Input: part model. Units: mm. Frame: model coordinates. Give positions to 0.01 mm unless a question says otherwise; leave off trailing zeros. Answer as a JSON object with one key per item and string values. Group by question number.
1) Ray query, L1, parallel to X at y = -0.9, z = -44; L2, parallel to Z at x = 123.5, y = -1.2; L3, parallel to Z at x = 13.5, y = -0.9. Return the intervals inside material, ascending.
2) First-contact query: P1, Ø1, axis at x = 26.5, y = -3.5, coming from the +Z side; P2, Ø1, axis at y = -2.5, z = -38.5, coming from the +X side; P3, Ø2, axis at y = -1.5, z = -44.5, coming from the -X side. Flat tips, straight axial feed; report the tip coordinate or a pass-through.
3) Section query A-A on y = -3.05. Count the separate pieces of the cut face and the enclosed holes in it, plus the area to 3 significant figures.
from build123d import *

# Parameters (mm, degrees)
F0_R     = 4.7625
F1_DEPTH = 4.7625
F2_R     = 5.08
F3_R     = 9.525
F4_R     = 0.381


with BuildPart() as f1:
    # F0 (on Front) → F1 (new body)
    with BuildSketch(Plane.XZ):
        with BuildLine():
            Line((60.1429268718, 16.5254306048), (-108.8427143228, -14.0530352161))
            Line((-108.8427143228, -14.0530352161), (-62.451031059, -57.4127137661))
            add(Edge.make_bspline(
                [(-62.451031059, -57.4127137661), (-50.1643598375, -47.5249055274), (10.3220797139, -17.4381564578), (123.773567881, 8.9901031394), (178.848968941, 3.3361169696)],
                knots=[0, 0, 0, 0, 0.398250962, 1, 1, 1, 1], degree=3))
            Line((178.848968941, 3.3361169696), (178.848968941, 52.8661169696))
            Line((178.848968941, 52.8661169696), (118.523968941, 52.8661169696))
            add(Edge.make_bspline(
                [(118.523968941, 52.8661169696), (115.1404463597, 48.2467955264), (112.3015113048, 24.068977806), (60.9008384489, 17.214194077), (60.1429268718, 16.5254306048)],
                knots=[0, 0, 0, 0, 0.4347885114, 1, 1, 1, 1], degree=3))
        make_face()
        with Locations((-43.4938967228, -22.9803621769)):
            Circle(F0_R, mode=Mode.SUBTRACT)
        with Locations((92.106996992, 10.612607679)):
            Circle(F0_R, mode=Mode.SUBTRACT)
    extrude(amount=F1_DEPTH)

    # F2
    f2_edges = [f1.edges().sort_by_distance(p)[0] for p in [
        (-62.451031, -2.38125, -57.412714),
        (178.848969, -2.38125, 3.336117),
    ]]
    fillet(f2_edges, radius=F2_R)

    # F3
    f3_edges = [f1.edges().sort_by_distance(p)[0] for p in [
        (-108.842714, -2.38125, -14.053035),
    ]]
    fillet(f3_edges, radius=F3_R)

    # F4
    f4_edges = [f1.edges().sort_by_distance(p)[0] for p in [
        (178.848969, -2.38125, 52.866117),
        (118.523969, -2.38125, 52.866117),
    ]]
    fillet(f4_edges, radius=F4_R)


solid = f1.part
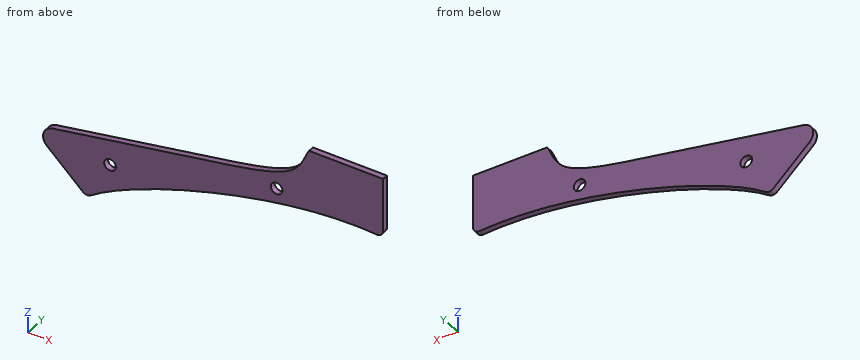
Output:
{
 "1": {"L1": "x = -76.8 to -40.89", "L2": "z = 2.86 to 52.87", "L3": "z = -21.71 to 8.09"},
 "2": {"P1": "stops at z = 10.53", "P2": "stops at x = -28.48", "P3": "stops at x = -77.34"},
 "3": {"separate pieces": "1", "enclosed holes": "2", "area": "9,790 mm^2"}
}
